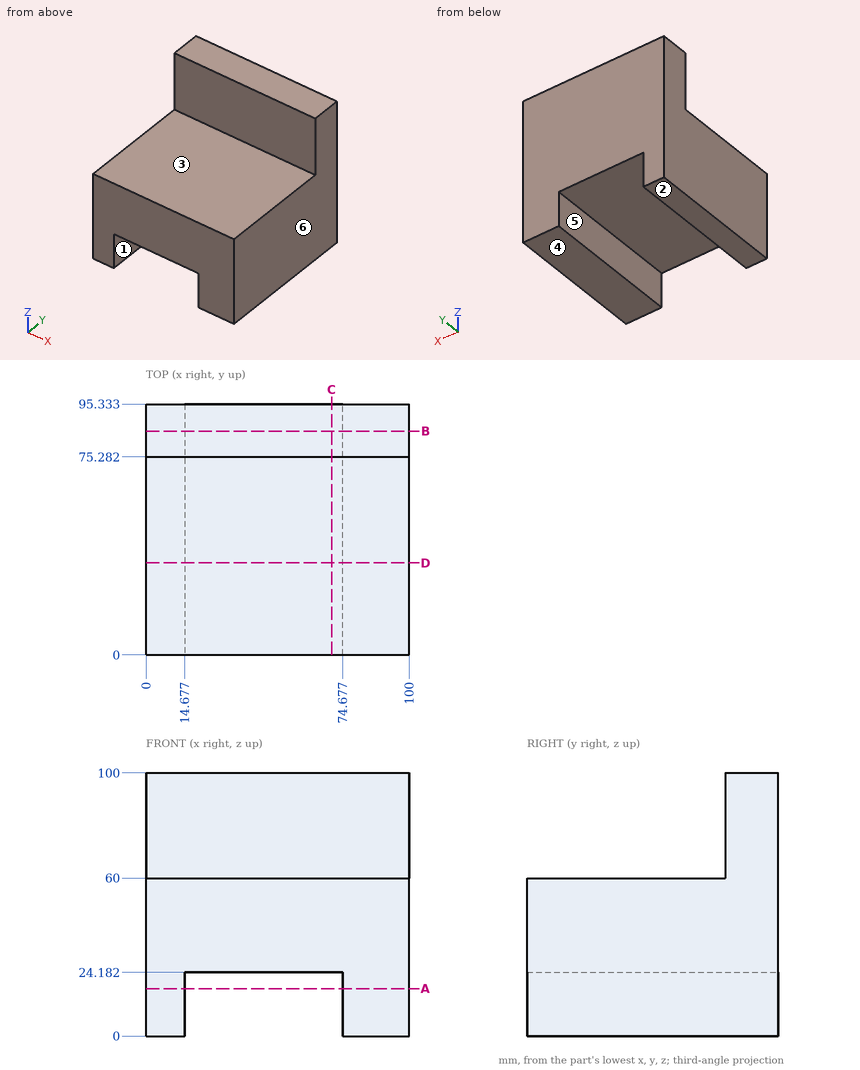
Part print with two shaded views. Sizes in mm from the minimum x, y, z corner. A direction names the side the tool comes from. Give positions to 0.01 mm unless a question says otherwise; leave off trailing zeros. Write each loop counter-clockwise with the first axis right and the second up, starting at its lowest first coordinate (ties: lowest second). Pieces come first, ordered by that corner, then holes.
1) Cut at C-C on x = 70.5. Write the cut outline in (y, z), then the cut area to 3 significant figures.
Resolved:
outline: (0, 24.18) - (95.33, 24.18) - (95.33, 100) - (75.28, 100) - (75.28, 60) - (0, 60) - close
area: 4,220 mm2
2) Cut at B-B on y = 85. Write the cut outline in (x, z).
Resolved:
outline: (0, 0) - (14.68, 0) - (14.68, 24.18) - (74.68, 24.18) - (74.68, 0) - (100, 0) - (100, 100) - (0, 100) - close
3) Pin check, flat tips, straight feed: pin 1 (20 mm diameter, centred on x = 39.5, z = 79.5, fed in from -Y); pin 2 (4 mm diameter, centred on x = 40, y = 40, fed in from -Z); pin 3 (10 mm diameter, centred on x = 26.5, y = 28.5, fed in from +Z). Stop position of each tip, or through.
Resolved:
pin 1: stops at y = 75.28
pin 2: stops at z = 24.18
pin 3: stops at z = 60
4) Two-plate mould, pull along X, no slides. Class the marked faces 4, 5 and 6: released by +X, released by -X, zero draft, split by the parting line, or undercut.
Resolved:
face 4: zero draft
face 5: undercut
face 6: released by +X
5) Cut at A-A on z = 18. Write the cut outline in (x, y).
Resolved:
outline: (0, 0) - (14.68, 0) - (14.68, 95.33) - (0, 95.33) - close; (74.68, 0) - (100, 0) - (100, 95.33) - (74.68, 95.33) - close
6) Probe L1, parallel to X at y = 13.5, z = 16; L2, parallel to Z at x = 79.5, y = 59; L3, parallel to Z at x = 66, y = 36.5. List the from-to ranges inside material, lowest first.
Resolved:
L1: x = 0 to 14.68, 74.68 to 100
L2: z = 0 to 60
L3: z = 24.18 to 60
7) Cut at D-D on y = 35. Write the cut outline in (x, z), then the cut area to 3 significant figures.
Resolved:
outline: (0, 0) - (14.68, 0) - (14.68, 24.18) - (74.68, 24.18) - (74.68, 0) - (100, 0) - (100, 60) - (0, 60) - close
area: 4,550 mm2
8) Which spindle directions (+Z, -Z, +X, -X, +Y, -Y) get a long thin tool onto all of the face, cutting with end or side? Do the marked faces 1, 2 and 3. Say none if no direction does.
Resolved:
face 1: -Z, +Y, -Y
face 2: -Z, +X, -X, +Y, -Y
face 3: +Z, +X, -X, -Y
